CAD build for the part. Positions are in the model's coordinates, mm. A direction names the side the tool comes from. Coordinates: 2 decimals unless noted, no trailing zeros. Write each loop counter-clockwise with the first axis right and the second up, starting at its lowest first coordinate (ties: lowest second). Pieces come first, ordered by that corner, then holes. Notation, with made-up numbers: (31, 58.25) - (81, 58.25) arc R26 cw to (81, 86.25) - close; hole circle Ø4 at (83, 82). An arc over 180 degrees is marked (long way). Answer in a Markdown table with one row per item. Add a question column.
Q1. Band-saw the part on C-C (x = 86). List the corners of the cut face in (y, z).
Q2. 3-axis set-ups, long thin cutter, end or side, ignore diameter. For faces 1 (the flat face through (-36, 11, 0)), 2 (the flat face through (-70.78, 145.01, 12.52)): which of +Z, -Z, +X, -X, +Y, -Y reach the whole face in a straight line?
Q3. Band-saw the part on D-D (x = 28.5). List the corners of the cut face in (y, z), and give its area (3 significant figures).
Q4. Two-plate mould, pull along X, no slides. Class faces 3 (the flat face through (-261.457, 45, 13)), 4 (the flat face through (30.82, 145.01, 12.52)), 5 (the flat face through (-36, -109.706, 13)): +X half, -X half, draft (parallel to the pull), parting line (faces both ways), or undercut.
Q5. Drill centre lines: line 1 along X through (y, z) = (124, 14.5); line 2 along X through (y, z) = (130, 2.5); line 3 along Y through (x, z) = (164, 4.25). Where is each one in solid material? Low to high. Write a range as from..to.
Q6. Band-saw the part on B-B (z = 8.25). List the corners of the cut face in (x, y).
Q7. Band-saw the part on A-A (y = 115). List the corners of the cut face in (x, z), and give its area (3 significant figures).
Q8. Pin check, flat tips, straight feed: pin 1 (1.5 mm diameter, centred on x = -49, z = 12.5, fed in from +Y); pin 2 (8 mm diameter, centred on x = 73, z = 14.5, fed in from +Y). Stop position of each tip, or through.
```python
from build123d import *

# Parameters (mm, degrees)
F1_DEPTH = 25.4


with BuildPart() as f1:
    # F0 (on Top) → F1 (new body)
    with BuildSketch(Plane.XY):
        Polygon((-261.456966, 195.094159), (-261.456966, -109.705841), (195.743034, -109.705841), (195.743034, 195.094159), (170.343034, 144.294159), (144.943034, 195.094159), (119.543034, 93.494159), (94.143034, 195.094159), (68.743034, 144.294159), (43.343034, 195.094159), (17.943034, 93.494159), (-7.456966, 195.094159), (-32.856966, 144.294159), (-58.256966, 195.094159), (-83.656966, 93.494159), (-109.056966, 195.094159), (-134.456966, 144.294159), (-159.856966, 195.094159), (-185.256966, 93.494159), (-210.656966, 195.094159), (-236.056966, 144.294159), align=None)
    extrude(amount=F1_DEPTH)


solid = f1.part
```
Checked values:
| question | item | result |
|---|---|---|
| 1 | outline | (-109.71, 0) - (178.81, 0) - (178.81, 25.4) - (-109.71, 25.4) - close |
| 2 | face 1 | -Z, +X, -X, +Y, -Y |
| 2 | face 2 | +Z, -Z, +Y |
| 3 | outline | (-109.71, 0) - (135.72, 0) - (135.72, 25.4) - (-109.71, 25.4) - close |
| 3 | area | 6,230 mm² |
| 4 | face 3 | -X half |
| 4 | face 4 | undercut |
| 4 | face 5 | draft |
| 5 | line 1 | x = -261.46..-192.88, -177.63..-91.28, -76.03..10.32, 25.57..111.92, 127.17..195.74 |
| 5 | line 2 | x = -261.46..-194.38, -176.13..-92.78, -74.53..8.82, 27.07..110.42, 128.67..195.74 |
| 5 | line 3 | y = -109.71..156.98 |
| 6 | outline | (-261.46, -109.71) - (195.74, -109.71) - (195.74, 195.09) - (170.34, 144.29) - (144.94, 195.09) - (119.54, 93.49) - (94.14, 195.09) - (68.74, 144.29) - (43.34, 195.09) - (17.94, 93.49) - (-7.46, 195.09) - (-32.86, 144.29) - (-58.26, 195.09) - (-83.66, 93.49) - (-109.06, 195.09) - (-134.46, 144.29) - (-159.86, 195.09) - (-185.26, 93.49) - (-210.66, 195.09) - (-236.06, 144.29) - (-261.46, 195.09) - close |
| 7 | outline | (-261.46, 0) - (-190.63, 0) - (-190.63, 25.4) - (-261.46, 25.4) - close; (-179.88, 0) - (-89.03, 0) - (-89.03, 25.4) - (-179.88, 25.4) - close; (-78.28, 0) - (12.57, 0) - (12.57, 25.4) - (-78.28, 25.4) - close; (23.32, 0) - (114.17, 0) - (114.17, 25.4) - (23.32, 25.4) - close; (124.92, 0) - (195.74, 0) - (195.74, 25.4) - (124.92, 25.4) - close |
| 7 | area | 10,500 mm² |
| 8 | pin 1 | stops at y = 178.08 |
| 8 | pin 2 | stops at y = 160.81 |
